Check sheet for the drawn part. Datum: minimum x, y, z corner. Units: mm. Coordinates: 2 decimals unless noted, no trailing zeros. Write each loop counter-clockwise with the first axis right and the second up, starting at its lowest first coordinate (ties: lowest second). Pieces come first, ordered by that corner, then holes. Notation, with made-up numbers: M 89.25,-3 L 123.25,-3 A23 cw 123.25,22 Z; hole C 22.25,3 d5. An arc over 180 degrees is marked long. Write item = value, one per line. Start each with the question number.
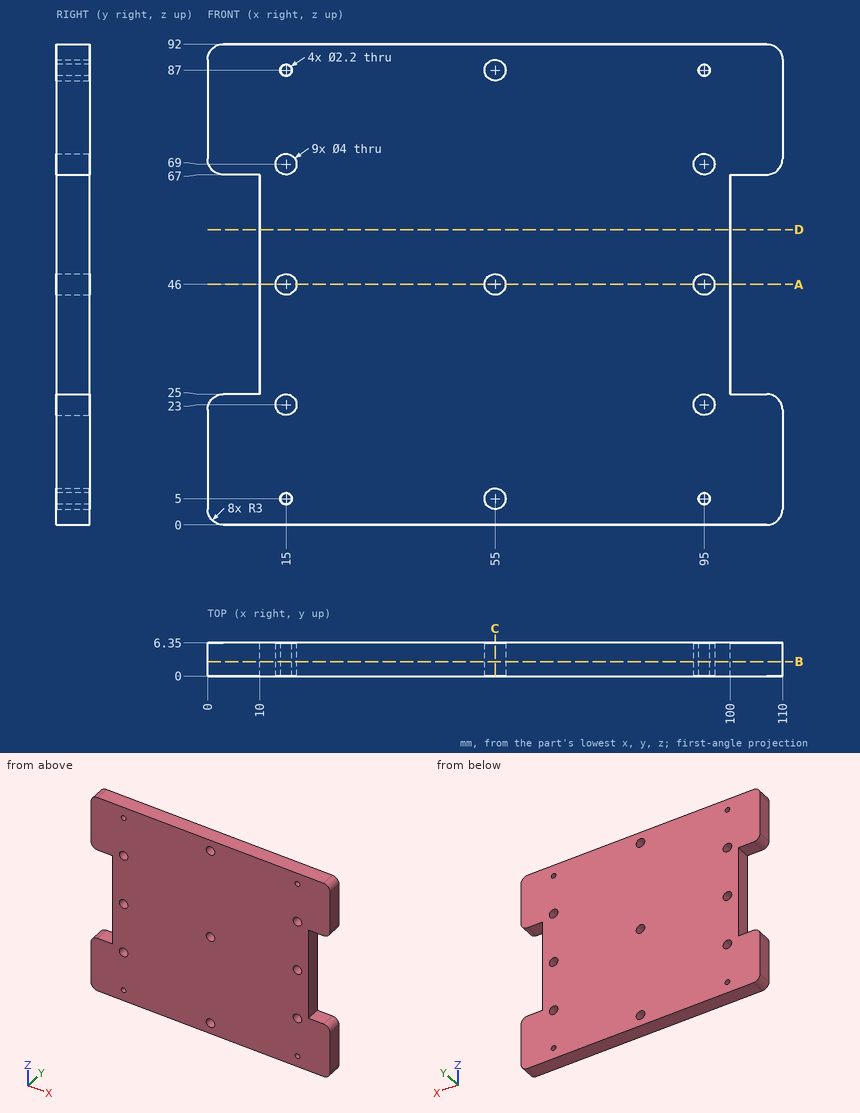
Q1. Cross-section at D-D on z = 56.5. Enter the section's corners in (x, y).
Q2. Cross-section at B-B on y = 2.75. Count the separate pieces of the cut face and the enclosed holes in it, and give its area (3 significant figures).
Q3. Cross-section at A-A on z = 46. Enter the section's corners in (x, y).
Q4. Gauge pin test, flat ends, axial feed: pin 1 (2 mm diameter, centred on y = 2.5, z = 68, fed in from -X); pin 2 (2.5 mm diameter, centred on x = 15, z = 69, fed in from -Y); pin 3 (1.5 mm diameter, centred on y = 4.5, z = 38, fed in from +X). Record the tip position at first contact, or that the pin passes through.
Q5. Scan lines: L1, parallel to Z at x = 15, y = 3.25; L2, parallel to X at y = 2.5, z = 46; L3, parallel to X at y = 3.5, z = 45. Record each from-to range of solid material in increasing order.
Q6. Cross-section at C-C on x = 55. Enter the section's corners in (y, z).
Values found:
q1.outline = M 10,0 L 100,0 L 100,6.35 L 10,6.35 Z
q2.separate_pieces = 1
q2.enclosed_holes = 13
q2.area = 9,140 mm²
q3.outline = M 10,0 L 13,0 L 13,6.35 L 10,6.35 Z; M 17,0 L 53,0 L 53,6.35 L 17,6.35 Z; M 57,0 L 93,0 L 93,6.35 L 57,6.35 Z; M 97,0 L 100,0 L 100,6.35 L 97,6.35 Z
q4.pin_1 = 0.17
q4.pin_2 = through
q4.pin_3 = 100
q5.L1 = 0 to 3.9, 6.1 to 21, 25 to 44, 48 to 67, 71 to 85.9, 88.1 to 92
q5.L2 = 10 to 13, 17 to 53, 57 to 93, 97 to 100
q5.L3 = 10 to 13.27, 16.73 to 53.27, 56.73 to 93.27, 96.73 to 100
q6.outline = M 0,0 L 6.35,0 L 6.35,3 L 0,3 Z; M 0,7 L 6.35,7 L 6.35,44 L 0,44 Z; M 0,48 L 6.35,48 L 6.35,85 L 0,85 Z; M 0,89 L 6.35,89 L 6.35,92 L 0,92 Z
